from build123d import *

# Parameters (mm, degrees)
SKETCH1_W          = 8.5
SKETCH1_H          = 201
SKETCH2_OUTSIDE_W  = 59.486
SKETCH2_OUTSIDE_H  = 59.486
SKETCH2_OUTSIDE_R  = 8
CUT_EXTRUDE1_DEPTH = 26
SKETCH3_W          = 3.25
SKETCH3_H          = 3.25
CUT_EXTRUDE2_DEPTH = 26
CHAMFER1_SIZE      = 0.5
SKETCH4_OUTSIDE_W  = 59.486
SKETCH4_OUTSIDE_H  = 59.486
SKETCH4_OUTSIDE_R  = 4
CUT_EXTRUDE3_DEPTH = 30
CHAMFER2_SIZE      = 1
SKETCH5_W          = 2.25
SKETCH5_H          = 2.25
CUT_EXTRUDE4_DEPTH = 30
CHAMFER3_SIZE      = 0.2


with BuildPart() as part:
    # Sketch1 → Revolve1 (revolve)
    with BuildSketch(Plane.XY, mode=Mode.PRIVATE) as revolve1_sk:
        with Locations((4.25, 100.5)):
            Rectangle(SKETCH1_W, SKETCH1_H)
    revolve(revolve1_sk.sketch.rotate(Axis((0, 201, 0), (0, -1, 0)), 180), axis=Axis((0, 201, 0), (0, -1, 0)))

    # Sketch2 outside → Cut-Extrude1 (cut)
    with BuildSketch(Plane(origin=(0, 201, 0), x_dir=(1, 0, 0), z_dir=(0, 1, 0))):
        Rectangle(SKETCH2_OUTSIDE_W, SKETCH2_OUTSIDE_H)
        with Locations(Location((0, 0, 0), (0, 0, 180))):
            Circle(SKETCH2_OUTSIDE_R, mode=Mode.SUBTRACT)
    extrude(amount=-CUT_EXTRUDE1_DEPTH, mode=Mode.SUBTRACT)

    # Sketch3 → Cut-Extrude2 (cut)
    with BuildSketch(Plane(origin=(0, 201, 0), x_dir=(1, 0, 0), z_dir=(0, 1, 0))):
        with Locations((0, 8)):
            Rectangle(SKETCH3_W, SKETCH3_H)
    extrude(amount=-CUT_EXTRUDE2_DEPTH, mode=Mode.SUBTRACT)

    # Chamfer1
    chamfer1_edges = [part.edges().sort_by_distance(p)[0] for p in [
        (0, 201, 8),
        (8.5, 0, 0),
    ]]
    chamfer(chamfer1_edges, length=CHAMFER1_SIZE)

    # Sketch4 outside → Cut-Extrude3 (cut)
    with BuildSketch(Plane.XZ):
        Rectangle(SKETCH4_OUTSIDE_W, SKETCH4_OUTSIDE_H)
        Circle(SKETCH4_OUTSIDE_R, mode=Mode.SUBTRACT)
    extrude(amount=-CUT_EXTRUDE3_DEPTH, mode=Mode.SUBTRACT)

    # Chamfer2
    chamfer2_edges = [part.edges().sort_by_distance(p)[0] for p in [
        (8.5, 30, 0),
    ]]
    chamfer(chamfer2_edges, length=CHAMFER2_SIZE)

    # Sketch5 → Cut-Extrude4 (cut)
    with BuildSketch(Plane.XZ):
        with Locations((0, 4)):
            Rectangle(SKETCH5_W, SKETCH5_H)
    extrude(amount=-CUT_EXTRUDE4_DEPTH, mode=Mode.SUBTRACT)

    # Chamfer3
    chamfer3_edges = [part.edges().sort_by_distance(p)[0] for p in [
        (0, 0, -4),
        (-1.125, 0, 3.356769067),
        (0, 0, 2.875),
        (1.125, 0, 3.356769067),
    ]]
    chamfer(chamfer3_edges, length=CHAMFER3_SIZE)


solid = part.part
For this review, take the finished solid that the model builds, in its own axes (mm). A direction names the side the tool comes from. Round coordinates to 2 decimals unless told otherwise and drop trailing zeros. Write each loop counter-clockwise with the first axis right and the second up, starting at its lowest first coordinate (ties: lowest second). Pieces come first, ordered by that corner, then holes. Notation, with made-up numbers: (49, 60) - (67, 60) arc R29 cw to (67, 85) - close; hole circle Ø1 at (33.5, 29.5). An arc over 180 degrees is marked (long way). Write item = value, one per line. Start each with the question number.
1. Draft analysis for pull direction X (two halves, no side actions). For faces 1 (the face through (0, 201, 0)), 2 (the face through (0, 188, -6.375)), 3 (the face through (0, 188, 8)), 4 (the face through (0, 175, -7)), state which applies: released by +X, released by -X, zero draft, split by the parting line, or undercut.
2. Consider section B-B on y = 15. State the section outline as (x, z) points (3 decimals).
3. Consider section D-D on y = 188. State the section outline as (x, z) points (3 decimals), plus the area to 3 significant figures.
4. For faces 5 (the face through (0.314, 200.865, 7.629)), 6 (the face through (0, 15, -4)), list the 3-axis set-ups (+Z, -Z, +X, -X, +Y, -Y) from which the entire face can be reached by the end or side of a thin tool; tool diameter is ignored.
5. Consider section C-C on y = 64.5. State the section outline as (x, z) points, plus the area to 3 significant figures.
6. Wall thickness on L1, parallel to X at y = 152.5, z = 0.75; L2, parallel to Z at x = 0.25, y = 25.5 (3 decimals); L3, parallel to Y at x = -4, z = -1.25: over which ranges is each line inside the solid? List them lowest first.
7. Consider section A-A on z = 0. State the section outline as (x, y) points.
8. For pin 1 Ø5 at (y, z) = (111.5, -0.5) entering from +X; pin 2 Ø4 at (y, z) = (35, -5.5) entering from +X; pin 3 Ø2.5 at (x, y) = (0.5, 185.5) entering from -Z; pin 4 Ø1.2 at (y, z) = (191, -7.5) entering from +X, all flat-tipped, find the tip position at first contact; note any pin that passes through.
Evaluation:
q1.face_1 = zero draft
q1.face_2 = undercut
q1.face_3 = split by the parting line
q1.face_4 = undercut
q2.outline = (-1.125, 2.875) - (-1.125, 3.839) arc R4 ccw (long way) to (1.125, 3.839) - (1.125, 2.875) - close
q3.outline = (-1.625, -7.833) - (-1.625, -6.375) - (1.625, -6.375) - (1.625, -7.833) arc R8 ccw (long way) to start
q3.area = 196 mm2
q4.face_5 = +Y
q4.face_6 = -Y
q5.outline = circle Ø17 at (0, 0)
q5.area = 227 mm2
q6.L1 = -8.47 to 8.47
q6.L2 = -3.992 to 2.875
q6.L3 = 30 to 201
q7.outline = (-8.5, 31) - (-7.5, 30) - (-4, 30) - (-4, 0.2) - (-3.8, 0) - (3.8, 0) - (4, 0.2) - (4, 30) - (7.5, 30) - (8.5, 31) - (8.5, 175) - (8, 175) - (8, 200.5) - (7.5, 201) - (-7.5, 201) - (-8, 200.5) - (-8, 175) - (-8.5, 175) - close
q8.pin_1 = 8.5
q8.pin_2 = 7.75
q8.pin_3 = -7.83
q8.pin_4 = 4.05
